```python
from build123d import *

# Parameters (mm, degrees)
EXTRUDE_1_DEPTH     = 3
EXTRUDE_2_DEPTH     = 3
CUT_EXTRUDE_1_DEPTH = 173.564004098


with BuildPart() as part:
    # 草图1 → 凸台-拉伸1 (new body)
    with BuildSketch(Plane(origin=(0, 0, 0), x_dir=(0, 0, -1), z_dir=(1, 0, 0))):
        with BuildLine():
            Line((-79.7507074, 150.000523308), (-49.751094174, 150.000523308))
            add(Edge.make_bspline(
                [(-49.751094174, 150.000523308), (0, 82.797016692), (49.751094174, 150.000523308)],
                knots=[0.222336685, 0.222336685, 0.222336685, 0.777663315, 0.777663315, 0.777663315], degree=2))
            Line((49.751094174, 150.000523308), (79.7507074, 150.000523308))
            add(Edge.make_bspline(
                [(-79.7507074, 150.000523308), (0, 22.797016692), (79.7507074, 150.000523308)],
                knots=[0.059549815, 0.059549815, 0.059549815, 0.940450185, 0.940450185, 0.940450185], degree=2))
        make_face()
    extrude(amount=EXTRUDE_1_DEPTH)

    # 草图2 → 凸台-拉伸2 (add)
    with BuildSketch(Plane(origin=(0, 150.000523308, 0), x_dir=(1, 0, 0), z_dir=(0, 1, 0))):
        Polygon((3, -59.750900787), (0.999993554, -59.750900787), (2.000006446, -69.750900787), (3, -69.750900787), align=None)
        Polygon((2.000006446, -69.750900787), (0.999993554, -59.750900787), (0, -59.750900787), (0, -69.750900787), align=None)
        Polygon((2.000006446, 59.750900787), (0.999993554, 69.750900787), (0, 69.750900787), (0, 59.750900787), align=None)
        Polygon((3, 69.750900787), (0.999993554, 69.750900787), (2.000006446, 59.750900787), (3, 59.750900787), align=None)
    extrude(amount=EXTRUDE_2_DEPTH)

    # 草图3 → 切除-拉伸1 (cut, through all)
    with BuildSketch(Plane.ZY):
        with BuildLine():
            Line((-1.5, 116.429314933), (-1.5, 99.990363817))
            Line((-1.5, 99.990363817), (1.5, 99.990363817))
            Line((1.5, 99.990363817), (1.5, 116.429314934))
            add(Edge.make_bspline(
                [(1.5, 116.429314934), (0, 116.368225067), (-1.5, 116.429314933)],
                knots=[0.491628426, 0.491628426, 0.491628426, 0.508371574, 0.508371574, 0.508371574], degree=2))
        make_face()
    extrude(amount=-CUT_EXTRUDE_1_DEPTH, mode=Mode.SUBTRACT)


solid = part.part
```
Part model, mm, in its own coordinate system. A direction names the side the tool comes from. Round coordinates to 2 decimals unless told otherwise and drop trailing zeros.
1. 3-axis set-ups, long thin cutter, end or side, ignore diameter. For faces 1 (the face through (1, 151, 69.751)), 2 (the face through (3, 117, -12)), 3 (the face through (1, 150.001, -75)), 4 (the face through (0, 117, -12)), 5 (the face through (1, 108, -1.5)): which of +Z, -Z, +X, -X, +Y, -Y reach the whole face in a straight line?
Solutions:
face 1: +Z, +X, -X, +Y
face 2: +Z, -Z, +X, +Y, -Y
face 3: -Z, +X, -X, +Y
face 4: +Z, -Z, -X, +Y, -Y
face 5: +X, -X, +Y
2. Flat gauge pins, fed straight in: pin 1 (0.9 mm diameter, centred on x = 1.5, z = 75.5, fed in from +Y); pin 2 (1.5 mm diameter, centred on x = 2, y = 151.5, fed in from -Z); pin 3 (1 mm diameter, centred on x = 1.5, z = -15, fed in from +Y). Where does each tip first touch, or does it go through?
Solutions:
pin 1: stops at y = 150
pin 2: stops at z = -69.75
pin 3: stops at y = 119.66
3. Drill centre lines: line 1 along Z through (x, y) = (1.75, 150.5); line 2 along Z through (x, y) = (0.55, 133); line 3 along Y through (x, z) = (1.7, 29.5). Where is each one in solid material? Low to high.
Solutions:
line 1: z = -69.75 to -59.75, 59.75 to 69.75
line 2: z = -68.27 to -34.97, 34.97 to 68.27
line 3: y = 95.1 to 128.21
